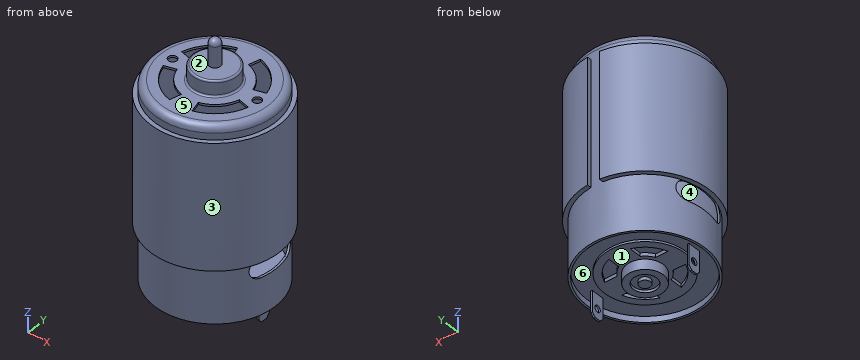
Autodesk Inventor part; units mm, degrees
ref_plane "Work Plane1" through (0, 0, -26.875) normal (0, 0, -1) x (-1, 0, 0)
ref_plane "Work Plane2" through (18, 0, 0) normal (1, 0, 0) x (0, 1, 0)
ref_plane "Work Plane3" through (0, 0, 24.625) normal (0, 0, 1) x (1, 0, 0)
sketch "Sketch1" plane through (0, 0, 0) normal (0, 0, 1) x (1, 0, 0)
  circle A0 centre (0, 0) radius 17.75
  dimension "d0" = 35.5
extrude "Extrusion1" add sketch "Sketch1" along normal mid plane 57.25
fillet "Fillet1" radius 2 1 edges at (-17.75, 0, 28.625)
shell "Shell1" thickness 0.62 removed faces 1 at (3.0438, 4.2648, -28.625)
sketch "Sketch2" plane through (0, 0, 28.625) normal (0, 0, 1) x (1, 0, 0)
  circle A0 centre (0, 0) radius 15.75
  circle A1 centre (0, 0) radius 6.5
  dimension "d5" = 13
extrude "Extrusion2" add sketch "Sketch2" along normal blind 4.5 contours A1
fillet "Fillet2" radius 0.5 2 edges at (-6.5, 0, 28.625) (-6.5, 0, 33.125)
sketch "Sketch3" plane through (0, 0, 33.125) normal (0, 0, 1) x (1, 0, 0)
  circle A0 centre (0, 0) radius 6
  circle A1 centre (0, 0) radius 1.6
  dimension "d9" = 3.2
extrude "Extrusion3" add sketch "Sketch3" along normal blind 7.62 contours A1
fillet "Fillet3" radius 1.6 1 edges at (-1.6, 0, 40.745)
sketch "Sketch4" plane through (0, 0, 28.625) normal (0, 0, 1) x (1, 0, 0)
  circle A0 centre (0, 0) radius 15.75
  point P0 (12.5, 0)
  dimension "d13" = 12.5
hole "Hole1" at (12.5, 0, 28.625) direction (0, 0, -1) diameter 2.5 depth 8 tip angle 118
mirror "Mirror1" about plane through (0, 0, 0) normal (1, 0, 0) of "Hole1"
sketch "Sketch5" plane through (0, 0, 28.625) normal (0, 0, 1) x (1, 0, 0)
  circle A0 centre (12.5, 0) radius 1.25
  circle A1 centre (0, 0) radius 7
  arc A2 (12.557, 3.3646) -> (3.3646, 12.557) centre (0, 0) ccw
  arc A3 (9.1763, 2.4588) -> (2.4588, 9.1763) centre (0, 0) ccw
  line L0 (0, 0) -> (3.3646, 12.557) construction
  line L1 (0, 0) -> (12.557, 3.3646) construction
  line L2 (2.4588, 9.1763) -> (3.3646, 12.557)
  line L3 (9.1763, 2.4588) -> (12.557, 3.3646)
  line L4 (0, 0) -> (12.5, 0) construction
  line L5 (0.151, 0.5634) -> (0.151, 14.7153) construction
  dimension "d21" = 15
  dimension "d22" = 15
  dimension "d23" = 13
  dimension "d24" = 9.5
extrude "Extrusion4" cut sketch "Sketch5" against normal blind 10 contours L3 A3 L2 A2
pattern_circular "Circular Pattern1" count 4 over 360 about axis through (0, 0, 0) along (0, 0, 1) of "Extrusion4"
ref_plane "Work Plane1" through (0, 0, -26.875) normal (0, 0, -1) x (-1, 0, 0)
sketch "Sketch6" plane through (0, 0, -26.875) normal (0, 0, -1) x (-1, 0, 0)
  circle A0 centre (0, 0) radius 17.13
extrude "Extrusion5" add sketch "Sketch6" against normal blind 0.62
sketch "Sketch7" plane through (0, 0, -26.875) normal (0, 0, -1) x (-1, 0, 0)
  circle A0 centre (0, 0) radius 17.13
  circle A1 centre (0, 0) radius 12
  dimension "d33" = 24
extrude "Extrusion6" add sketch "Sketch7" along normal blind 0.62 contours A1
sketch "Sketch8" plane through (0, 0, -27.495) normal (0, 0, -1) x (-1, 0, 0)
  circle A0 centre (0, 0) radius 12
  circle A1 centre (0, 0) radius 5.375
  dimension "d36" = 10.75
extrude "Extrusion7" add sketch "Sketch8" along normal blind 3 contours A1
sketch "Sketch9" plane through (0, 0, -30.495) normal (0, 0, -1) x (-1, 0, 0)
  circle A0 centre (0, 0) radius 5.375
  circle A1 centre (0, 0) radius 3.45
  dimension "d39" = 6.9
extrude "Extrusion8" cut sketch "Sketch9" against normal blind 0.8 contours A1
sketch "Sketch10" plane through (0, 0, -29.695) normal (0, 0, -1) x (-1, 0, 0)
  circle A0 centre (0, 0) radius 3.45
  circle A1 centre (0, 0) radius 1.6
  dimension "d42" = 3.2
extrude "Extrusion9" add sketch "Sketch10" along normal blind 1 contours A1
sketch "Sketch11" plane through (0, 0, -27.495) normal (0, 0, -1) x (-1, 0, 0)
  circle A0 centre (0, 0) radius 5.375
  circle A1 centre (0, 0) radius 12
  arc A2 (9.3591, 3.15) -> (3.15, 9.3591) centre (0, 0) ccw
  arc A3 (5.6857, 3.15) -> (3.15, 5.6857) centre (0, 0) ccw
  line L0 (3.15, 9.3591) -> (3.15, 5.6857)
  line L1 (5.6857, 3.15) -> (9.3591, 3.15)
  dimension "d45" = 3.15
  dimension "d46" = 3.15
  dimension "d47" = 9.875
  dimension "d48" = 6.5
extrude "Extrusion10" cut sketch "Sketch11" against normal blind 1 contours L1 A3 L0 A2
pattern_circular "Circular Pattern2" count 4 over 360 about axis through (0, 0, 0) along (0, 0, 1) of "Extrusion10"
sketch "Sketch12" plane through (0, 0, -26.875) normal (0, 0, -1) x (-1, 0, 0)
  circle A0 centre (0, 0) radius 12
  circle A1 centre (0, 0) radius 17.13
  line L0 (-14.5, 1.9) -> (-14, 1.9)
  line L1 (-14, 1.9) -> (-14, -1.9)
  line L2 (-14, -1.9) -> (-14.5, -1.9)
  line L3 (-14.5, -1.9) -> (-14.5, 1.9)
  line L4 (0, 0) -> (-16.9017, 0) construction
  point P0 (-14, 0)
  dimension "d54" = 0.5
  dimension "d55" = 3.8
  dimension "d56" = 14
extrude "Extrusion11" add sketch "Sketch12" along normal blind 7.2 contours L0 L1 L2 L3
chamfer "Chamfer1" distance 1 angle 45 2 edges at (14.25, 1.9, -34.075) (14.25, -1.9, -34.075)
sketch "Sketch13" plane through (14.5, -1.9, -26.875) normal (1, 0, 0) x (0, 0, -1)
  line L0 (7.2, 1) -> (7.2, 2.8)
  line L1 (4.2, 1.9) -> (6.2, 3.8) construction
  line L2 (4.2, 1.9) -> (6.2, 0) construction
  dimension "d61" = 3
hole "Hole2" at (14.5, 0, -31.075) direction (-1, 0, 0) diameter 2 depth 1 tip angle 118
mirror "Mirror2" about plane through (0, 0, 0) normal (1, 0, 0) of "Extrusion11", "Chamfer1", "Hole2"
ref_plane "Work Plane2" through (18, 0, 0) normal (1, 0, 0) x (0, 1, 0)
sketch "Sketch14" plane through (18, 0, 0) normal (1, 0, 0) x (0, 1, 0)
  arc A0 (-4.5554, -11.975) -> (-4.5554, -17.875) centre (-4.5554, -14.925) ccw
  arc A1 (5.2946, -17.875) -> (5.2946, -11.975) centre (5.2946, -14.925) ccw
  line L0 (-4.5554, -11.975) -> (5.2946, -11.975)
  line L1 (-4.5554, -17.875) -> (5.2946, -17.875)
  line L2 (17.75, -28.625) -> (-17.75, -28.625)
  line L3 (0, -28.625) -> (0, 20.5314) construction
  dimension "d70" = 10.75
  dimension "d71" = 5.9
  dimension "d72" = 9.85
extrude "Extrusion12" cut sketch "Sketch14" against normal through all
ref_plane "Work Plane3" through (0, 0, 24.625) normal (0, 0, 1) x (1, 0, 0)
sketch "Sketch15" plane through (0, 0, 24.625) normal (0, 0, 1) x (1, 0, 0)
  circle A0 centre (0, 0) radius 17.75
  arc A1 (-1.75, 18.9192) -> (1.75, 18.9192) centre (0, 0) ccw
  line L0 (-1.75, 18.9192) -> (-1.75, 17.6635)
  line L1 (1.75, 18.9192) -> (1.75, 17.6635)
  line L2 (0, 0) -> (0, 21.9354) construction
  dimension "d76" = 38
  dimension "d77" = 3.5
extrude "Extrusion13" add sketch "Sketch15" against normal blind 37 contours A0 L1 A1 L0
properties part number "FisherPriceMotor" material "ABS Plastic"
The model under review builds one solid part; all positions refer to its coordinate system, in mm. Face numbers are marked on the shaded views. A direction names the side the tool comes from. Give positions to 0.01 mm unless a question says otherwise; leave off trailing zeros. Write each loop counter-clockwise with the first axis right and the second up, starting at its lowest first coordinate (ties: lowest second). Pieces come first, ordered by that corner, then holes. Notation, with made-up numbers: (-4, -24) -> (4, -24) arc R25 ccw to (4, -9) -> close; hole circle Ø6 at (-20, -13.5). An arc over 180 degrees is marked (long way). Put each result on its own line as item: value.
(1) We need section D-D, the plane z = 2.5. Give the boundary of the cut face in (x, y), and give its area (3 significant figures).
Results are:
outline: (-1.75, 17.66) -> (-1.75, 18.92) arc R19 ccw (long way) to (1.75, 18.92) -> (1.75, 17.66) arc R17.75 ccw to start; hole circle Ø34.26 at (0, 0)
area: 208 mm²
(2) The part is to be moulded in two halves that separate along Z. For the marked faces 3, 4, 5 and 6, say which applies: pulls with the +Z half, pulls with the -Z half, needs draft (parallel to the pull), parting line crosses it, or undercut.
Results are:
face 3: needs draft
face 4: undercut
face 5: pulls with the +Z half
face 6: pulls with the -Z half
(3) To check wall thickness, follow probe 1 along Y at (x, z) = (0, -29.95) (3 decimals); probe 2 along Z at (x, y) = (14.2, 0) (3 decimals); probe 3 along Z at (x, y) = (6.5, -5.5) (3 decimals). State the ranges of each line that lie inside material, in increasing order. Write a range as from..to.
Results are:
probe 1: -5.375..-3.45, -1.6..1.6, 3.45..5.375
probe 2: -34.075..-32.075, -30.075..-26.255, 28.005..28.625
probe 3: -26.495..-26.255, 28.005..28.625
(4) We need section A-A, the plane z = -24.5. Give the boundary of the cut face in (x, y), and give its area (3 significant figures).
Results are:
outline: circle Ø35.5 at (0, 0); hole circle Ø34.26 at (0, 0)
area: 67.9 mm²
(5) We need section B-B, the plane y = 0. State how many separate pieces and enclosed holes the cut face has, and give its area (3 significant figures).
Results are:
separate pieces: 6
enclosed holes: 0
area: 326 mm²
(6) We need section C-C, the plane z = 31. Give the boundary of the cut face in (x, y).
Results are:
outline: circle Ø13 at (0, 0)
(7) For pin 1 Ø1 at (x, y) = (4.5, -7) entering from +Z (3 decimals); pin 2 Ø1.4 at (y, z) = (18, 12.5) entering from +X; pin 3 Ø1.5 at (y, z) = (-7.5, 14) entering from -X, all flat-tipped, find the tip position at first contact; note any pin that passes through.
Results are:
pin 1: z = 28.625
pin 2: x = 7.86
pin 3: x = -17.76
(8) Tool access review of the marked faces 1 and 2: name each direction out of +Z, -Z, +X, -X, +Y, -Y from which nothing blocks a thin tool from reaching the whole face with its end or side.
Results are:
face 1: -Z
face 2: +Z
